from build123d import *

# Parameters (mm, degrees)
SKETCH_R     = 2.75
PAD_DEPTH    = 10
FILLET_R     = 1
CHAMFER_SIZE = 1
SKETCH001_R  = 5
POCKET_DEPTH = 5


with BuildPart() as part:
    # Sketch → Pad (new body)
    with BuildSketch(Plane.XY):
        with BuildLine():
            ThreePointArc((0, 7.5), (-7.5, 0), (0, -7.5))
            Line((0, -7.5), (15, -7.5))
            ThreePointArc((15, -7.5), (22.5, 0), (15, 7.5))
            Line((0, 7.5), (15, 7.5))
        make_face()
        Circle(SKETCH_R, mode=Mode.SUBTRACT)
        with Locations((15, 0)):
            Circle(SKETCH_R, mode=Mode.SUBTRACT)
    extrude(amount=PAD_DEPTH)

    # Fillet
    fillet_edges = [part.edges().sort_by_distance(p)[0] for p in [
        (7.5, -7.5, 10),
    ]]
    fillet(fillet_edges, radius=FILLET_R)

    # Chamfer
    chamfer_edges = [part.edges().sort_by_distance(p)[0] for p in [
        (12.25, 0, 0),
        (-2.75, 0, 0),
    ]]
    chamfer(chamfer_edges, length=CHAMFER_SIZE)

    # Sketch001 (on Face14 of Chamfer) → Pocket (cut)
    with BuildSketch(Plane.XY.offset(10)):
        Circle(SKETCH001_R)
        with Locations((15, 0)):
            Circle(SKETCH001_R)
    extrude(amount=-POCKET_DEPTH, mode=Mode.SUBTRACT)


solid = part.part
Verification items for the finished model (mm, model axes). A direction names the side the tool comes from. Coordinates: 2 decimals unless noted, no trailing zeros. Order: outer loops, then holes, each group sorted by start corner. A loop starts at its lowest first (then second) coordinate and runs counter-clockwise, first axis right, second up.
1. Release check for a two-part mould opening along X. For faces 3 (the face through (19.77, 1.5, 7.54)), 4 (the face through (22.5, -0.16, 4.44)), 5 (the face through (-7.5, 0.16, 4.44)), 6 (the face through (7.605, -7.215, 9.699)) record: +X half, -X half, draft (parallel to the pull), parting line (faces both ways), or undercut.
Results found:
face 3: undercut
face 4: +X half
face 5: -X half
face 6: draft
2. Sectioned sample at A-A, the plane y = 0. Record the cut outline in (x, z), and give its area (3 significant figures).
Results found:
outline: (-7.5, 0) - (-3.75, 0) - (-2.75, 1) - (-2.75, 5) - (-5, 5) - (-5, 10) - (-6.5, 10) arc R1 ccw to (-7.5, 9) - close; (2.75, 1) - (3.75, 0) - (11.25, 0) - (12.25, 1) - (12.25, 5) - (10, 5) - (10, 10) - (5, 10) - (5, 5) - (2.75, 5) - close; (17.75, 1) - (18.75, 0) - (22.5, 0) - (22.5, 9) arc R1 ccw to (21.5, 10) - (20, 10) - (20, 5) - (17.75, 5) - close
area: 143 mm2
3. Go/stop test with flat-tipped pins: pin 1 Ø1.5 at (y, z) = (-1, 1.5) entering from -X; pin 2 Ø1 at (y, z) = (1.5, 5) entering from +X; pin 3 Ø3 at (x, y) = (2.5, 2) entering from +Z. Record where each tip stops, or that it passes through.
Results found:
pin 1: stops at x = -7.5
pin 2: stops at x = 22.43
pin 3: stops at z = 5
4. Sectioned sample at D-D, the plane y = -2. Give the number of separate pieces and of enclosed holes in the cut face, and give its area (3 significant figures).
Results found:
separate pieces: 3
enclosed holes: 0
area: 162 mm2
5. Scan lines: line 1 (X direction, y = 0, z = 2.15); line 2 (Y direction, x = 15, z = 7.8); line 3 (Y direction, x = 0, z = 2.4). Record each from-to range of solid material in increasing order.
Results found:
line 1: x = -7.5 to -2.75, 2.75 to 12.25, 17.75 to 22.5
line 2: y = -7.5 to -5, 5 to 7.5
line 3: y = -7.5 to -2.75, 2.75 to 7.5
6. Sectioned sample at B-B, the plane z = 3.25. Record the cut outline in (x, y).
Results found:
outline: (0, -7.5) - (15, -7.5) arc R7.5 ccw to (15, 7.5) - (0, 7.5) arc R7.5 ccw to start; hole circle Ø5.5 at (0, 0); hole circle Ø5.5 at (15, 0)
7. Sectioned sample at C-C, the plane z = 9.5. Record the cut outline in (x, y).
Results found:
outline: (0, -7.37) - (15, -7.37) arc R7.37 ccw to (15, 7.37) - (0, 7.37) arc R7.37 ccw to start; hole circle Ø10 at (0, 0); hole circle Ø10 at (15, 0)
8. Set-up check for faces 1 (the face through (2.2, -2.2, 5)), 2 (the face through (-0.596, -2.685, 2.972)): record each of +Z, -Z, +X, -X, +Y, -Y from which the full face is reachable in a straight line by a thin tool's end or side.
Results found:
face 1: +Z
face 2: +Z, -Z
